Check sheet for the modelled part. Datum: model origin and axes. Units: mm. Give positions to 0.01 mm unless a question says otherwise; leave off trailing zeros. Loops run counter-clockwise (first coordinate to the right, second up) from the corner with the lowest first, then second, coordinate; pieces in that order, holes last. Notation, with made-up numbers: M 4,-3 L 42,-3 A9 cw 42,10 Z; hole C 67,-35.5 d8. An arc over 180 degrees is marked long. One line per question, with ' | ' between items. Start each with the question number.
from build123d import *

# Parameters (mm, degrees)
SKETCH1_R                   = 21.59
BASE_FLANGE1_DEPTH          = 3.03784
F_11_0_191_DIAMETER_HOLE1_D = 4.8514
F_11_0_191_DIAMETER_HOLE2_D = 4.8514


# Sheet-metal steps are written as plain solids
with BuildPart() as part:
    # Sketch1 → Base-Flange1 (new body)
    with BuildSketch(Plane(origin=(0, 0, 0), x_dir=(1, 0, 0), z_dir=(0, 1, 0))):
        with BuildLine():
            Line((9.946664741, 0), (498.053335259, 0))
            ThreePointArc((498.053335259, 0), (503.405631357, 2.933067681), (503.813471801, 9.022700323))
            Line((503.813471801, 9.022700323), (300.081092338, 448.101602582))
            ThreePointArc((300.081092338, 448.101602582), (254, 477.52), (207.918907662, 448.101602582))
            Line((207.918907662, 448.101602582), (4.186528199, 9.022700323))
            ThreePointArc((4.186528199, 9.022700323), (4.594368643, 2.933067681), (9.946664741, 0))
        make_face()
        with Locations(Location((254, 426.72, 0), (0, 0, 270))):
            Circle(SKETCH1_R, mode=Mode.SUBTRACT)
    extrude(amount=-BASE_FLANGE1_DEPTH)

    # #11 (0.191) Diameter Hole1 (through all)
    with Locations(Plane(origin=(0, 0, 0), x_dir=(1, 0, 0), z_dir=(0, 1, 0))):
        with Locations((61.947885367, 47.625), (87.347885367, 47.625), (112.747885367, 47.625), (228.6, 47.625), (254, 47.625), (446.052114633, 47.625), (420.652114633, 47.625), (395.252114633, 47.625), (279.4, 47.625), (103.499910638, 177.8), (114.190711929, 200.840546169), (124.88151322, 223.881092338), (404.500089362, 177.8), (393.809288071, 200.840546169), (383.11848678, 223.881092338)):
            Hole(F_11_0_191_DIAMETER_HOLE1_D / 2)

    # #11 (0.191) Diameter Hole2 (through all)
    with Locations(Plane(origin=(0, 0, 0), x_dir=(1, 0, 0), z_dir=(0, 1, 0))):
        with Locations((228.6, 386.588000012), (254, 386.588000012), (279.4, 386.588000012)):
            Hole(F_11_0_191_DIAMETER_HOLE2_D / 2)


solid = part.part
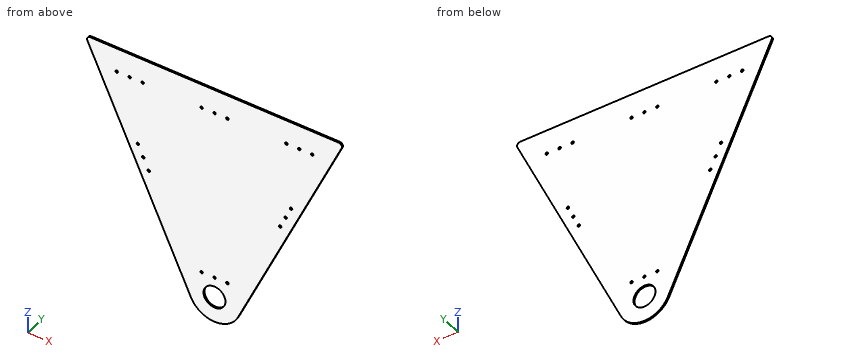
Q1. Material ranges on probe 1 along Z at (x, y) = (228.6, -1.9); probe 2 along X at (y, z) = (-1.7, -226); probe 3 along X at (y, z) = (-2.6, -241), recorded low to high. Write a range as from..to.
Q2. Cross-section at C-C (x = 148). Record the cut outline in (y, z), and give its area (3 significant figures).
Q3. Cross-section at A-A (z = -426.72). Record the cut outline in (x, y), and give its area (3 significant figures).
Q4. Depth check by flat-ended pin: P1, Ø1.5, axis at x = 197.5, y = -2, coming from the -Z side. Enter the tip coordinate at first touch or a pass-through.
Q5. Cross-section at B-B (y = -2.1). State how many separate pieces and enclosed holes the cut face has, and give its area (3 significant figures).
Q6. Cross-section at D-D (z = -270). Record the cut outline in (x, y), and give its area (3 significant figures).
Solved:
1) probe 1: z = -470.71..-389.01, -384.16..-50.05, -45.2..0 | probe 2: x = 104.86..123.7, 126.06..381.94, 384.3..403.14 | probe 3: x = 111.82..396.18
2) outline: M -3.04,-318.97 L 0,-318.97 L 0,0 L -3.04,0 Z | area: 969 mm²
3) outline: M 198,-3.04 L 232.41,-3.04 L 232.41,0 L 198,0 Z; M 275.59,-3.04 L 310,-3.04 L 310,0 L 275.59,0 Z | area: 209 mm²
4) P1: stops at z = -427.26
5) separate pieces: 1 | enclosed holes: 19 | area: 135,000 mm²
6) outline: M 125.28,-3.04 L 382.72,-3.04 L 382.72,0 L 125.28,0 Z | area: 782 mm²
